CAD build for the part. Positions are in the model's coordinates, mm. Round coordinates to 2 decimals unless told otherwise and drop trailing zeros.
from build123d import *

# Parameters (mm, degrees)
SKETCH1_W                 = 308.11216
SKETCH1_H                 = 3.175
BOSS_EXTRUDE1_DEPTH       = 267.83
SKETCH3_W                 = 267.83
SKETCH3_H                 = 3.175
BOSS_EXTRUDE3_DEPTH       = 3.175
SKETCH4_W                 = 50.87366
SKETCH4_H                 = 3.175
BOSS_EXTRUDE4_DEPTH       = 267.83
CUT_EXTRUDE1_DEPTH        = 340.191055801
CUT_EXTRUDE3_DEPTH        = 340.191055801
SKETCH19_R                = 5
CUT_EXTRUDE5_DEPTH        = 340.191055801
LPATTERN1_COUNT           = 3
LPATTERN1_PITCH           = 11
LPATTERN2_COUNT           = 3
LPATTERN2_PITCH           = 11
LPATTERN2_COPY_1_SKETCH_R = 5
LPATTERN2_COPY_1_DEPTH    = 340.191055801
LPATTERN2_COPY_2_SKETCH_R = 5
LPATTERN2_COPY_2_DEPTH    = 340.191055801
LPATTERN2_COPY_3_SKETCH_R = 5
LPATTERN2_COPY_3_DEPTH    = 340.191055801
LPATTERN2_COPY_4_SKETCH_R = 5
LPATTERN2_COPY_4_DEPTH    = 340.191055801
LPATTERN3_COUNT           = 2
LPATTERN3_PITCH           = 66
LPATTERN3_COPY_1_SKETCH_R = 5
LPATTERN3_COPY_1_DEPTH    = 340.191055801
LPATTERN3_COPY_2_SKETCH_R = 5
LPATTERN3_COPY_2_DEPTH    = 340.191055801
LPATTERN3_COPY_3_SKETCH_R = 5
LPATTERN3_COPY_3_DEPTH    = 340.191055801
LPATTERN3_COPY_4_SKETCH_R = 5
LPATTERN3_COPY_4_DEPTH    = 340.191055801
LPATTERN3_COPY_5_SKETCH_R = 5
LPATTERN3_COPY_5_DEPTH    = 340.191055801
LPATTERN3_COPY_6_SKETCH_R = 5
LPATTERN3_COPY_6_DEPTH    = 340.191055801
LPATTERN3_COPY_7_SKETCH_R = 5
LPATTERN3_COPY_7_DEPTH    = 340.191055801
LPATTERN3_COPY_8_SKETCH_R = 5
LPATTERN3_COPY_8_DEPTH    = 340.191055801
SKETCH21_W                = 105.9343525
SKETCH21_H                = 3.175
BOSS_EXTRUDE5_DEPTH       = 3.175
CUT_EXTRUDE9_DEPTH        = 340.191055801
CUT_EXTRUDE9_DEPTH_BACK   = 340.191055801
CUT_EXTRUDE11_DEPTH       = 340.191055801
CUT_EXTRUDE11_DEPTH_BACK  = 80.645
SKETCH32_R                = 3
M4_CLEARANCE_HOLE1_D      = 4.5
SKETCH35_W                = 80
SKETCH35_H                = 3.1635
BOSS_EXTRUDE6_DEPTH       = 3.175
SKETCH36_R                = 2.4
CUT_EXTRUDE12_DEPTH       = 340.191055801
LPATTERN4_COUNT           = 3
LPATTERN4_PITCH           = 58


with BuildPart() as part:
    # Sketch1 → Boss-Extrude1 (new body)
    with BuildSketch(Plane.XY):
        Rectangle(SKETCH1_W, SKETCH1_H)
    extrude(amount=BOSS_EXTRUDE1_DEPTH)

    # Sketch3 → Boss-Extrude3 (add)
    with BuildSketch(Plane(origin=(154.05608, 0, 0), x_dir=(0, 0, -1), z_dir=(1, 0, 0))):
        with Locations((-133.915, 0)):
            Rectangle(SKETCH3_W, SKETCH3_H)
    extrude(amount=BOSS_EXTRUDE3_DEPTH)

    # Sketch4 → Boss-Extrude4 (add)
    with BuildSketch(Plane.XY.offset(267.83)):
        with Locations((182.66791, 0)):
            Rectangle(SKETCH4_W, SKETCH4_H)
    extrude(amount=-BOSS_EXTRUDE4_DEPTH)

    # Sketch6 → Cut-Extrude1 (cut, through all)
    with BuildSketch(Plane(origin=(0, 1.5875, 0), x_dir=(1, 0, 0), z_dir=(0, 1, 0))):
        Polygon((208.10474, -240.606362049), (106.50474, -267.83), (208.10474, -267.83), align=None)
    extrude(amount=-CUT_EXTRUDE1_DEPTH, mode=Mode.SUBTRACT)

    # Sketch11 → Cut-Extrude3 (cut, through all)
    with BuildSketch(Plane.XZ.offset(1.5875)):
        Polygon((-154.05608, 242.43), (-84.20608, 267.83), (-154.05608, 267.83), align=None)
    extrude(amount=-CUT_EXTRUDE3_DEPTH, mode=Mode.SUBTRACT)

    # Sketch19 → Cut-Extrude5 (cut, through all)
    with BuildSketch(Plane(origin=(0, 1.5875, 0), x_dir=(1, 0, 0), z_dir=(0, 1, 0))):
        with Locations(Location((172.48674, -49.774823778, 0), (0, 0, 270))):
            Circle(SKETCH19_R)
    cut_extrude5 = extrude(amount=-CUT_EXTRUDE5_DEPTH, mode=Mode.SUBTRACT)

    # LPattern1: Cut-Extrude5 ×3
    with Locations(*[(i * LPATTERN1_PITCH, 0, 0) for i in range(1, LPATTERN1_COUNT)]):
        add(cut_extrude5, mode=Mode.SUBTRACT)

    # LPattern2: Cut-Extrude5 ×3
    with Locations(*[(0, 0, i * LPATTERN2_PITCH) for i in range(1, LPATTERN2_COUNT)]):
        add(cut_extrude5, mode=Mode.SUBTRACT)

    # LPattern2 copy 1 sketch → LPattern2 copy 1 (cut, through all)
    with BuildSketch(Plane(origin=(11, 1.5875, 11), x_dir=(1, 0, 0), z_dir=(0, 1, 0))):
        with Locations(Location((172.48674, -49.774823778, 0), (0, 0, 270))):
            Circle(LPATTERN2_COPY_1_SKETCH_R)
    extrude(amount=-LPATTERN2_COPY_1_DEPTH, mode=Mode.SUBTRACT)

    # LPattern2 copy 2 sketch → LPattern2 copy 2 (cut, through all)
    with BuildSketch(Plane(origin=(11, 1.5875, 22), x_dir=(1, 0, 0), z_dir=(0, 1, 0))):
        with Locations(Location((172.48674, -49.774823778, 0), (0, 0, 270))):
            Circle(LPATTERN2_COPY_2_SKETCH_R)
    extrude(amount=-LPATTERN2_COPY_2_DEPTH, mode=Mode.SUBTRACT)

    # LPattern2 copy 3 sketch → LPattern2 copy 3 (cut, through all)
    with BuildSketch(Plane(origin=(22, 1.5875, 11), x_dir=(1, 0, 0), z_dir=(0, 1, 0))):
        with Locations(Location((172.48674, -49.774823778, 0), (0, 0, 270))):
            Circle(LPATTERN2_COPY_3_SKETCH_R)
    extrude(amount=-LPATTERN2_COPY_3_DEPTH, mode=Mode.SUBTRACT)

    # LPattern2 copy 4 sketch → LPattern2 copy 4 (cut, through all)
    with BuildSketch(Plane(origin=(22, 1.5875, 22), x_dir=(1, 0, 0), z_dir=(0, 1, 0))):
        with Locations(Location((172.48674, -49.774823778, 0), (0, 0, 270))):
            Circle(LPATTERN2_COPY_4_SKETCH_R)
    extrude(amount=-LPATTERN2_COPY_4_DEPTH, mode=Mode.SUBTRACT)

    # LPattern3: Cut-Extrude5 ×2
    with Locations(*[(0, 0, i * LPATTERN3_PITCH) for i in range(1, LPATTERN3_COUNT)]):
        add(cut_extrude5, mode=Mode.SUBTRACT)

    # LPattern3 copy 1 sketch → LPattern3 copy 1 (cut, through all)
    with BuildSketch(Plane(origin=(11, 1.5875, 66), x_dir=(1, 0, 0), z_dir=(0, 1, 0))):
        with Locations(Location((172.48674, -49.774823778, 0), (0, 0, 270))):
            Circle(LPATTERN3_COPY_1_SKETCH_R)
    extrude(amount=-LPATTERN3_COPY_1_DEPTH, mode=Mode.SUBTRACT)

    # LPattern3 copy 2 sketch → LPattern3 copy 2 (cut, through all)
    with BuildSketch(Plane(origin=(22, 1.5875, 66), x_dir=(1, 0, 0), z_dir=(0, 1, 0))):
        with Locations(Location((172.48674, -49.774823778, 0), (0, 0, 270))):
            Circle(LPATTERN3_COPY_2_SKETCH_R)
    extrude(amount=-LPATTERN3_COPY_2_DEPTH, mode=Mode.SUBTRACT)

    # LPattern3 copy 3 sketch → LPattern3 copy 3 (cut, through all)
    with BuildSketch(Plane(origin=(0, 1.5875, 77), x_dir=(1, 0, 0), z_dir=(0, 1, 0))):
        with Locations(Location((172.48674, -49.774823778, 0), (0, 0, 270))):
            Circle(LPATTERN3_COPY_3_SKETCH_R)
    extrude(amount=-LPATTERN3_COPY_3_DEPTH, mode=Mode.SUBTRACT)

    # LPattern3 copy 4 sketch → LPattern3 copy 4 (cut, through all)
    with BuildSketch(Plane(origin=(0, 1.5875, 88), x_dir=(1, 0, 0), z_dir=(0, 1, 0))):
        with Locations(Location((172.48674, -49.774823778, 0), (0, 0, 270))):
            Circle(LPATTERN3_COPY_4_SKETCH_R)
    extrude(amount=-LPATTERN3_COPY_4_DEPTH, mode=Mode.SUBTRACT)

    # LPattern3 copy 5 sketch → LPattern3 copy 5 (cut, through all)
    with BuildSketch(Plane(origin=(11, 1.5875, 77), x_dir=(1, 0, 0), z_dir=(0, 1, 0))):
        with Locations(Location((172.48674, -49.774823778, 0), (0, 0, 270))):
            Circle(LPATTERN3_COPY_5_SKETCH_R)
    extrude(amount=-LPATTERN3_COPY_5_DEPTH, mode=Mode.SUBTRACT)

    # LPattern3 copy 6 sketch → LPattern3 copy 6 (cut, through all)
    with BuildSketch(Plane(origin=(11, 1.5875, 88), x_dir=(1, 0, 0), z_dir=(0, 1, 0))):
        with Locations(Location((172.48674, -49.774823778, 0), (0, 0, 270))):
            Circle(LPATTERN3_COPY_6_SKETCH_R)
    extrude(amount=-LPATTERN3_COPY_6_DEPTH, mode=Mode.SUBTRACT)

    # LPattern3 copy 7 sketch → LPattern3 copy 7 (cut, through all)
    with BuildSketch(Plane(origin=(22, 1.5875, 77), x_dir=(1, 0, 0), z_dir=(0, 1, 0))):
        with Locations(Location((172.48674, -49.774823778, 0), (0, 0, 270))):
            Circle(LPATTERN3_COPY_7_SKETCH_R)
    extrude(amount=-LPATTERN3_COPY_7_DEPTH, mode=Mode.SUBTRACT)

    # LPattern3 copy 8 sketch → LPattern3 copy 8 (cut, through all)
    with BuildSketch(Plane(origin=(22, 1.5875, 88), x_dir=(1, 0, 0), z_dir=(0, 1, 0))):
        with Locations(Location((172.48674, -49.774823778, 0), (0, 0, 270))):
            Circle(LPATTERN3_COPY_8_SKETCH_R)
    extrude(amount=-LPATTERN3_COPY_8_DEPTH, mode=Mode.SUBTRACT)

    # Sketch21 → Boss-Extrude5 (add)
    with BuildSketch(Plane.ZY.offset(154.05608)):
        with Locations((189.46282375, 0)):
            Rectangle(SKETCH21_W, SKETCH21_H)
    extrude(amount=BOSS_EXTRUDE5_DEPTH)

    # Sketch27 → Cut-Extrude9 (cut, two sides: drawn at the far end of the back side and taken through both)
    with BuildSketch(Plane(origin=(0, 1.5875, 0), x_dir=(1, 0, 0), z_dir=(0, 1, 0)).offset(-CUT_EXTRUDE9_DEPTH_BACK)):
        Polygon((748.107746333, -570.489573212), (-84.20608, -267.83), (-154.05608, -242.43), (-157.23108, -241.275454545), (-989.544906333, 61.384118666), (-1594.864052757, -1603.243534), (142.788599909, -2235.117225879), align=None)
    extrude(amount=CUT_EXTRUDE9_DEPTH + CUT_EXTRUDE9_DEPTH_BACK, mode=Mode.SUBTRACT)

    # Sketch32 → Cut-Extrude11 (cut, two sides: drawn at the far end of the back side and taken through both)
    with BuildSketch(Plane(origin=(0, 1.5875, 0), x_dir=(1, 0, 0), z_dir=(0, 1, 0)).offset(-CUT_EXTRUDE11_DEPTH_BACK)):
        with Locations(Location((172.54426, -240.761310541, 0), (0, 0, 90))):
            Circle(SKETCH32_R)
        with Locations(Location((131.90426, -252.445254824, 0), (0, 0, 90))):
            Circle(SKETCH32_R)
        with Locations(Location((73.48426, -258.94, 0), (0, 0, 90))):
            Circle(SKETCH32_R)
        with Locations(Location((11.25426, -258.94, 0), (0, 0, 90))):
            Circle(SKETCH32_R)
        with Locations(Location((-50.97574, -258.94, 0), (0, 0, 90))):
            Circle(SKETCH32_R)
        with Locations(Location((-115.3206, -247.915394364, 0), (0, 0, 90))):
            Circle(SKETCH32_R)
    extrude(amount=CUT_EXTRUDE11_DEPTH + CUT_EXTRUDE11_DEPTH_BACK, mode=Mode.SUBTRACT)

    # M4 Clearance Hole1 (through all)
    with Locations(Plane(origin=(0, 1.5875, 0), x_dir=(1, 0, 0), z_dir=(0, 1, 0))):
        with Locations((180.96500002, -180.586), (105.42905, -212.2849914), (3.82905, -212.2849914), (-97.77095, -212.2849914)):
            Hole(M4_CLEARANCE_HOLE1_D / 2)

    # Sketch35 → Boss-Extrude6 (add)
    with BuildSketch(Plane(origin=(0, 0, 0), x_dir=(-1, 0, 0), z_dir=(0, 0, -1))):
        with Locations((-2.78399998, 0.00575)):
            Rectangle(SKETCH35_W, SKETCH35_H)
    extrude(amount=BOSS_EXTRUDE6_DEPTH)

    # Sketch36 → Cut-Extrude12 (cut, symmetric)
    with BuildSketch(Plane(origin=(0, 1.5875, 0), x_dir=(1, 0, 0), z_dir=(0, 1, 0))):
        with Locations(Location((183.48674, -35.774823778, 0), (0, 0, 270))):
            Circle(SKETCH36_R)
    cut_extrude12 = extrude(amount=CUT_EXTRUDE12_DEPTH, both=True, mode=Mode.SUBTRACT)

    # LPattern4: Cut-Extrude12 ×3
    with Locations(*[(0, 0, i * LPATTERN4_PITCH) for i in range(1, LPATTERN4_COUNT)]):
        add(cut_extrude12, mode=Mode.SUBTRACT)


solid = part.part
Item 1: Wall check: L1, parallel to Z at x = -51, y = -0.4; L2, parallel to X at y = -1.25, z = 68; L3, parallel to X at y = -1.1, z = 53. Give the ranges that are in metal, low to high.
Verdict:
L1: z = 0 to 255.94, 261.94 to 267.83
L2: x = -154.06 to 169.21, 175.77 to 180.21, 186.77 to 191.21, 197.77 to 208.1
L3: x = -154.06 to 168.67, 176.31 to 179.67, 187.31 to 190.67, 198.31 to 208.1
Item 2: Mould opens along X. For faces 1 (the flat face through (158.016, 0.022, 254.028)), 2 (the flat face through (28, 1.588, 130)), 3 (the cylindrical face through (199.444, 0.022, 49.124)) say: released by +X, released by -X, zero draft, split by the parting line, or undercut.
Verdict:
face 1: released by +X
face 2: zero draft
face 3: undercut
Item 3: Flat gauge pins, fed straight in: P1, Ø9, axis at x = 183.49, z = 137.77, coming from the +Y side; P2, Ø1, axis at x = 21, z = -1.5, coming from the -Y side; P3, Ø0.9, axis at y = 0, z = -2, coming from the -X side; P4, Ø11.5, axis at x = 172.49, z = 126.77, coming from the +Y side. Where does each tip first touch, or does it go through?
Verdict:
P1: passes through
P2: stops at y = -1.58
P3: stops at x = -37.22
P4: stops at y = 1.59
Item 4: Cut at A-A (y = -0.6). State how many separate pieces and enclosed holes the cut face has, plus the area to 3 significant figures.
Verdict:
separate pieces: 1
enclosed holes: 31
area: 93,600 mm2
